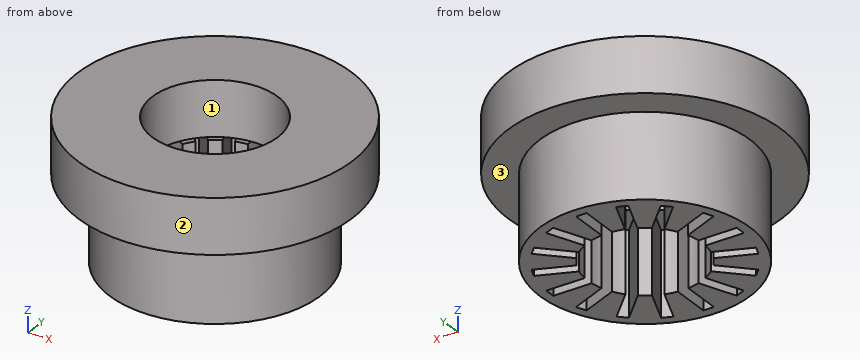
from build123d import *

# Parameters (mm, degrees)
SKETCH006_R   = 13
SKETCH006_R_2 = 5.95
PAD003_DEPTH  = 5.2
SKETCH_R      = 10
SKETCH_R_2    = 5.45
PAD_DEPTH     = 8
SKETCH002_W   = 1
SKETCH002_H   = 18.16
SKETCH002_W_2 = 18.16
SKETCH002_H_2 = 1
POCKET_DEPTH  = 13


with BuildPart() as linear_bearing_holder:
    # Sketch006 → Pad003 (new body)
    with BuildSketch(Plane.XY):
        Circle(SKETCH006_R)
        Circle(SKETCH006_R_2, mode=Mode.SUBTRACT)
    extrude(amount=PAD003_DEPTH)


with BuildPart() as linearbearingfusion:
    # Sketch → Pad (new body)
    with BuildSketch(Plane.XY):
        Circle(SKETCH_R)
        Circle(SKETCH_R_2, mode=Mode.SUBTRACT)
    extrude(amount=PAD_DEPTH)

    # Sketch002 → Pocket (cut)
    with BuildSketch(Plane.XY):
        Rectangle(SKETCH002_W, SKETCH002_H)
        Polygon((3.015215, 8.578896), (-3.940517, -8.197161), (-3.016771, -8.580167), (3.938961, 8.19589), align=None)
        Polygon((6.056348, 6.770742), (-6.77744, -6.049612), (-6.070703, -6.757089), (6.763084, 6.063266), align=None)
        Polygon((8.203481, 3.930131), (-8.582606, -3.005738), (-8.200729, -3.929951), (8.585358, 3.005918), align=None)
        with Locations((0.000556, -0.009993)):
            Rectangle(SKETCH002_W_2, SKETCH002_H_2)
        Polygon((8.585358, -3.005918), (-8.191917, 3.970918), (-8.57589, 3.047573), (8.201385, -3.929262), align=None)
        Polygon((6.763084, -6.063266), (-6.042956, 6.783069), (-6.751173, 6.077074), (6.054867, -6.769261), align=None)
        Polygon((3.938961, -8.19589), (-2.974592, 8.585961), (-3.899205, 8.205052), (3.014349, -8.576799), align=None)
    extrude(amount=POCKET_DEPTH, mode=Mode.SUBTRACT)


with BuildPart() as linearbearingfusion_1:
    # Body placement: moved
    add(linearbearingfusion.part.moved(Location((0, 0, -8))))

    # Fusion002: union linear_bearing_holder
    add(linear_bearing_holder.part)


with BuildPart() as linearbearingfusion_2:
    # Fusion002 placement: moved
    add(linearbearingfusion_1.part.moved(Location((0, 0, -5))))


solid = linearbearingfusion_2.part
Source: CAD feature listing. Evaluate the final solid. Frame: model axes, mm. Face numbers are marked on the shaded views. A direction names the side the tool comes from. Give positions to 0.01 mm unless a question says otherwise; leave off trailing zeros. Write each loop counter-clockwise with the first axis right and the second up, starting at its lowest first coordinate (ties: lowest second). Pieces come first, ordered by that corner, then holes. Notation, with made-up numbers: M 88,32 L 138,32 A11 ccw 138,41 Z; hole C 44.25,34 d5. An arc over 180 degrees is marked long. Return JSON: item names as keys, results as strings. Group by question number.
1) Material intervals for line 1 along Y through (x, z) = (0, -1.65); line 2 along X through (y, z) = (6, -6); line 3 along X through (y, z) = (-3.25, -12), sorted ascending. Write a range as [from, to].
2) Pin query (flat end, axial travel): P1, Ø0.6, axis at x = 4.5, y = 3, coming from the +Z side; P2, Ø3, axis at y = 0.5, z = -11, coming from the +X side; P3, Ø1.1, axis at y = 7, z = -7.5, coming from the -X side. Return the tip coordinate at first contact, or that it passes through.
3) Set-up query: the marked faces 1, 2 and 3. Return all of +Z, -Z, +X, -X, +Y, -Y with unobstructed straight access to the full face (end or side cutting, diameter ignored); none if empty.
4) Cut plane C-C, the plane z = -2.25. Output: boundary loops of the cut face in (x, y), plus the area to 3 significant figures.
5) Cut plane D-D, the plane y = 7.5. Output: boundary loops of the cut face in (x, z), plus the area to 3 significant figures.
6) Cut plane A-A, the plane y = 0. Output: boundary loops of the cut face in (x, z).
Recorded:
{
 "1": {"line 1": "y = [-13, -5.95], [5.95, 13]", "line 2": "x = [-8, -6.67], [-5.26, -2.99], [-1.91, -0.5], [0.5, 1.95], [3.03, 5.28], [6.7, 8]", "line 3": "x = [-9.46, -8.48], [-6.56, -4.37], [4.37, 6.57], [8.48, 9.46]"},
 "2": {"P1": "stops at z = -5", "P2": "stops at x = 10", "P3": "stops at x = -7.64"},
 "3": {"face 1": "+Z", "face 2": "+Z, -Z", "face 3": "-Z"},
 "4": {"outline": "C 0,0 d26; hole C 0,0 d11.9", "area": "420 mm²"},
 "5": {"outline": "M -10.62,-5 L -6.61,-5 L -6.61,-13 L -3.61,-13 L -3.61,-5 L -2.53,-5 L -2.53,-13 L -0.5,-13 L -0.5,-5 L 0.5,-5 L 0.5,-13 L 2.57,-13 L 2.57,-5 L 3.65,-5 L 3.65,-13 L 6.61,-13 L 6.61,-5 L 10.62,-5 L 10.62,0.2 L -10.62,0.2 Z", "area": "191 mm²"},
 "6": {"outline": "M -13,-5 L -10,-5 L -10,-13 L -9.08,-13 L -9.08,-5 L -5.95,-5 L -5.95,0.2 L -13,0.2 Z; M 5.95,-5 L 9.08,-5 L 9.08,-13 L 10,-13 L 10,-5 L 13,-5 L 13,0.2 L 5.95,0.2 Z"}
}
